Here's the drawing with two shaded views (mm, measured from the low corner). I have some questions. A direction names the side the tool comes from. Coordinates: 2 decimals unless noted, no trailing zeros. Loops run counter-clockwise (first coordinate to the right, second up) from the corner with the lowest first, then second, coordinate; pieces in that order, holes last.
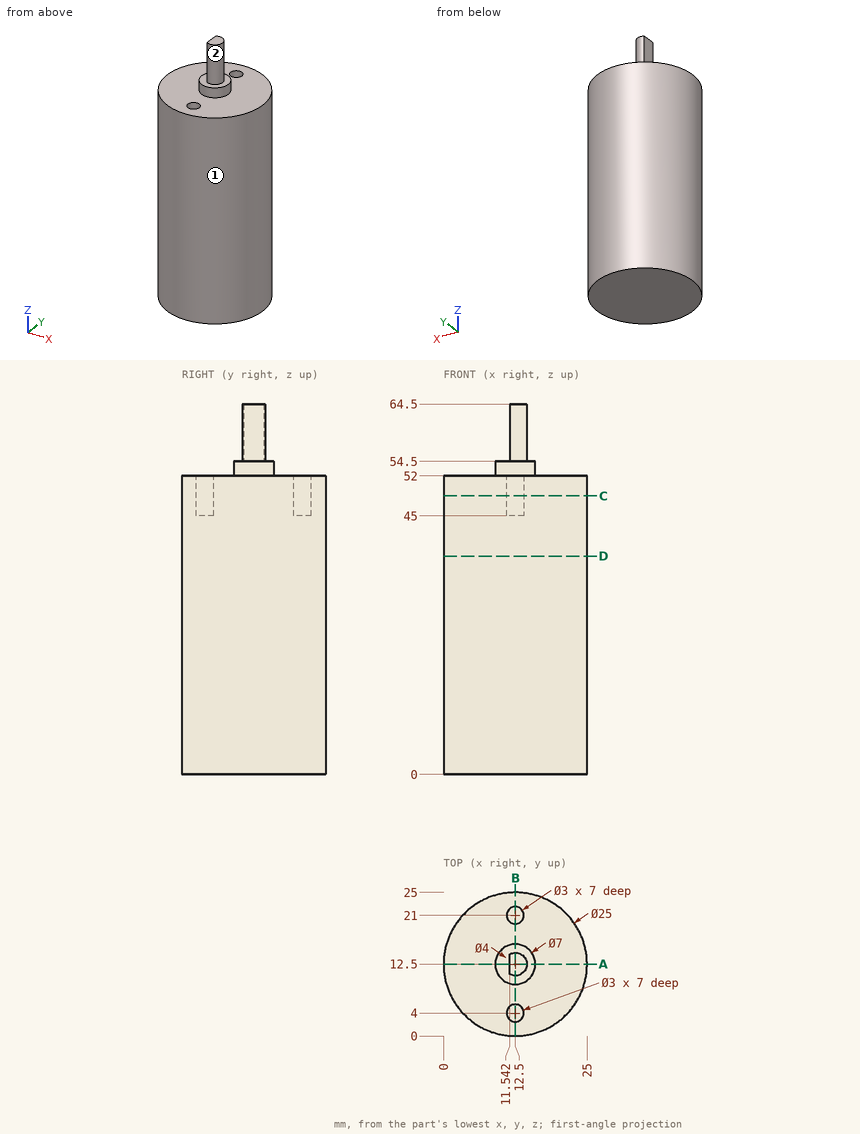
Q1. Suppose I cut it at B-B on x = 12.5. Write out the boundary of the cut face in (y, z).
Q2. Suppose I cut it at A-A on y = 12.5. Write out the boundary of the cut face in (x, z), and give its area (3 significant figures).
Q3. For the marked faces 1 and 2, which set-ups out of +Z, -Z, +X, -X, +Y, -Y let a thin tool reach every point of the face, with its end or its side?
Q4. Please list where these lines run through material, in increasing order: probe 1 along Y at (x, z) = (12.5, 48.5); probe 2 along Z at (x, y) = (2, 8); probe 3 along X at (y, z) = (12.25, 47).
Q5. Suppose I cut it at D-D on z = 38. Write out the boundary of the cut face in (x, y).
Q6. Will these pins go through, and if not, where does the flat tip stop? P1, Ø1.8, axis at y = 12.5, z = 58, coming from the -X side; P2, Ø3, axis at y = 20.5, z = 52, coming from the +X side; P3, Ø8, axis at x = 22, z = 34, coming from the -Y side (3 decimals); P4, Ø7.5, axis at x = 14.5, y = 9, coming from the +Z side.
Q7. Suppose I cut it at C-C on z = 48.5. Write out the boundary of the cut face in (x, y), and give its area (3 significant figures).
Check values:
1. outline: (0, 0) - (25, 0) - (25, 52) - (22.5, 52) - (22.5, 45) - (19.5, 45) - (19.5, 52) - (16, 52) - (16, 54.5) - (14.5, 54.5) - (14.5, 64.5) - (10.5, 64.5) - (10.5, 54.5) - (9, 54.5) - (9, 52) - (5.5, 52) - (5.5, 45) - (2.5, 45) - (2.5, 52) - (0, 52) - close
2. outline: (0, 0) - (25, 0) - (25, 52) - (16, 52) - (16, 54.5) - (14.5, 54.5) - (14.5, 64.5) - (11.54, 64.5) - (11.54, 54.5) - (9, 54.5) - (9, 52) - (0, 52) - close
2. area: 1,350 mm2
3. face 1: +Z, -Z
3. face 2: +Z
4. probe 1: y = 0 to 2.5, 5.5 to 19.5, 22.5 to 25
4. probe 2: z = 0 to 52
4. probe 3: x = 0 to 25
5. outline: circle Ø25 at (12.5, 12.5)
6. P1: stops at x = 11.54
6. P2: stops at x = 23.18
6. P3: stops at y = 1.275
6. P4: stops at z = 64.5
7. outline: circle Ø25 at (12.5, 12.5); hole circle Ø3 at (12.5, 4); hole circle Ø3 at (12.5, 21)
7. area: 477 mm2
